Source: CAD feature listing. Evaluate the final solid. Frame: model axes, mm. A direction names the side the tool comes from. Coordinates: 2 decimals unless noted, no trailing zeros. Write each loop counter-clockwise with the first axis right and the second up, starting at its lowest first coordinate (ties: lowest second). Pieces come first, ordered by that corner, then holes. Notation, with made-up numbers: (62, 5) - (80, 5) arc R27 cw to (80, 29) - close; hole circle Ø11 at (29, 59). An arc over 180 degrees is marked (long way). One line per item, written item: value.
from build123d import *

# Parameters (mm, degrees)
CROQUIS1_R              = 1.5
CROQUIS1_W              = 23
CROQUIS1_H              = 10.5
CROQUIS1_R_2            = 1.55
CROQUIS1_W_2            = 8
CROQUIS1_H_2            = 24
SALIENTE_EXTRUIR1_DEPTH = 1


with BuildPart() as part:
    # Croquis1 → Saliente-Extruir1 (new body)
    with BuildSketch(Plane.XY):
        with BuildLine():
            ThreePointArc((309.850726744, 63.509654663), (309.599394258, 62.624115136), (309.514659431, 61.707508197))
            Line((309.514659431, 61.707508197), (309.514659431, 57.327552176))
            ThreePointArc((309.514659431, 57.327552176), (303.729213281, 45.491505651), (290.835726452, 42.785700432))
            ThreePointArc((290.835726452, 42.785700432), (280.128411441, 45.991903753), (269.737322706, 50.109136972))
            ThreePointArc((269.737322706, 50.109136972), (267.74260814, 50.759780707), (265.656038098, 50.97989188))
            Line((265.656038098, 50.97989188), (241.08166038, 50.97989188))
            ThreePointArc((241.08166038, 50.97989188), (235.230334816, 49.089268499), (231.591539837, 44.13228971))
            ThreePointArc((231.591539837, 44.13228971), (233.256794927, -20.949922712), (276.095054953, -69.973905885))
            ThreePointArc((276.095054953, -69.973905885), (277.267588571, -70.441900659), (278.519966502, -70.601286078))
            Line((278.519966502, -70.601286078), (293.924380078, -70.601286078))
            Line((293.924380078, -70.601286078), (366.696152251, -70.601286078))
            ThreePointArc((366.696152251, -70.601286078), (367.948530182, -70.441900659), (369.121063801, -69.973905885))
            ThreePointArc((369.121063801, -69.973905885), (412.002341733, -20.83942385), (413.549540259, 44.357259338))
            ThreePointArc((413.549540259, 44.357259338), (409.908538666, 49.29800924), (404.067243855, 51.18140435))
            Line((404.067243855, 51.18140435), (380.008708846, 51.18140435))
            ThreePointArc((380.008708846, 51.18140435), (377.904907933, 50.95760104), (375.895274543, 50.296208695))
            ThreePointArc((375.895274543, 50.296208695), (365.751190215, 46.2242243), (355.299933141, 43.021923672))
            ThreePointArc((355.299933141, 43.021923672), (342.343405641, 45.666690288), (336.514525798, 57.536423018))
            Line((336.514525798, 57.536423018), (336.514525798, 61.707508197))
            ThreePointArc((336.514525798, 61.707508197), (336.429790971, 62.624115136), (336.178458485, 63.509654663))
            ThreePointArc((336.178458485, 63.509654663), (323.014592614, 72.53553857), (309.850726744, 63.509654663))
        make_face()
        with Locations((256.640896295, -50.101286078)):
            Circle(CROQUIS1_R, mode=Mode.SUBTRACT)
        with Locations((293.924380078, -67.101286078)):
            Circle(CROQUIS1_R, mode=Mode.SUBTRACT)
        with BuildLine():
            Line((287.201459209, -57.50788535), (267.201459209, -57.50788535))
            ThreePointArc((267.201459209, -57.50788535), (277.201459209, -47.50788535), (287.201459209, -57.50788535))
        make_face(mode=Mode.SUBTRACT)
        Polygon((259.608059377, -32.937061776), (253.608059377, -32.937061776), (253.608059377, -12.437061776), (265.608059377, -12.437061776), (265.608059377, -32.937061776), align=None, mode=Mode.SUBTRACT)
        with BuildLine():
            Line((250.731722484, 10.184978786), (250.731722484, -19.815021214))
            Line((250.731722484, -19.815021214), (238.731722484, -19.815021214))
            ThreePointArc((238.731722484, -19.815021214), (238.55388558, -2.343886452), (250.731722484, 10.184978786))
        make_face(mode=Mode.SUBTRACT)
        with Locations((260.608059377, -4.351286077)):
            Circle(CROQUIS1_R, mode=Mode.SUBTRACT)
        with BuildLine():
            ThreePointArc((301.108080537, -22.687061776), (304.239766137, -32.687061776), (301.108080537, -42.687061776))
            Line((301.108080537, -42.687061776), (272.308080537, -42.687061776))
            ThreePointArc((272.308080537, -42.687061776), (269.176394936, -32.687061776), (272.308080537, -22.687061776))
            ThreePointArc((272.308080537, -22.687061776), (286.708080537, -18.980626962), (301.108080537, -22.687061776))
        make_face(mode=Mode.SUBTRACT)
        with Locations((311.80644959, -22.701286077)):
            Circle(CROQUIS1_R, mode=Mode.SUBTRACT)
        with Locations((322.608059377, -22.701286077)):
            Circle(CROQUIS1_R, mode=Mode.SUBTRACT)
        with Locations((311.80644959, -16.851286077)):
            Circle(CROQUIS1_R, mode=Mode.SUBTRACT)
        with Locations((322.608059377, -16.851286077)):
            Circle(CROQUIS1_R, mode=Mode.SUBTRACT)
        with BuildLine():
            Line((331.039483308, -59.416197143), (322.608059377, -67.00788535))
            Line((322.608059377, -67.00788535), (314.115647223, -59.484458572))
            Line((314.115647223, -59.484458572), (308.293872865, -60.935989946))
            Line((308.293872865, -60.935989946), (305.497908348, -56.790802083))
            ThreePointArc((305.497908348, -56.790802083), (297.524016311, -57.967163869), (290.57468702, -62.050496292))
            ThreePointArc((290.57468702, -62.050496292), (296.700568728, -48.781397839), (309.575833339, -41.865983052))
            Line((309.575833339, -41.865983052), (317.608059377, -45.629378016))
            ThreePointArc((317.608059377, -45.629378016), (317.926050133, -44.19732179), (318.644984002, -42.91863604))
            Line((318.644984002, -42.91863604), (318.642820451, -42.911559385))
            Line((318.642820451, -42.911559385), (317.961360482, -40.68260426))
            Line((317.961360482, -40.68260426), (320.108059377, -42.359789251))
            Line((320.108059377, -42.359789251), (322.608059377, -42.359789251))
            Line((322.608059377, -42.359789251), (325.108059377, -42.359789251))
            Line((325.108059377, -42.359789251), (327.254758271, -40.68260426))
            Line((327.254758271, -40.68260426), (326.573298302, -42.911559385))
            Line((326.573298302, -42.911559385), (326.571134752, -42.91863604))
            ThreePointArc((326.571134752, -42.91863604), (327.29006862, -44.19732179), (327.608059377, -45.629378016))
            Line((327.608059377, -45.629378016), (334.361262908, -41.934506878))
            ThreePointArc((334.361262908, -41.934506878), (348.087721137, -48.396503366), (354.701459209, -62.050496292))
            ThreePointArc((354.701459209, -62.050496292), (347.70490498, -57.902513314), (339.657222183, -56.722540654))
            Line((339.657222183, -56.722540654), (336.861257666, -60.867728516))
            Line((336.861257666, -60.867728516), (331.039483308, -59.416197143))
        make_face(mode=Mode.SUBTRACT)
        with Locations((351.291980078, -67.101286078)):
            Circle(CROQUIS1_R, mode=Mode.SUBTRACT)
        with BuildLine():
            ThreePointArc((358.014659544, -57.50788535), (368.014659544, -47.50788535), (378.014659544, -57.50788535))
            Line((378.014659544, -57.50788535), (358.014659544, -57.50788535))
        make_face(mode=Mode.SUBTRACT)
        with Locations((388.037027296, -50.101286078)):
            Circle(CROQUIS1_R, mode=Mode.SUBTRACT)
        with Locations((322.608059377, -32.75788535)):
            Rectangle(CROQUIS1_W, CROQUIS1_H, mode=Mode.SUBTRACT)
        with Locations((333.505439463, -22.701286077)):
            Circle(CROQUIS1_R, mode=Mode.SUBTRACT)
        with BuildLine():
            ThreePointArc((372.908059377, -22.687061776), (376.039744977, -32.687061776), (372.908059377, -42.687061776))
            Line((372.908059377, -42.687061776), (344.108059377, -42.687061776))
            ThreePointArc((344.108059377, -42.687061776), (340.976373776, -32.687061776), (344.108059377, -22.687061776))
            ThreePointArc((344.108059377, -22.687061776), (358.508059377, -18.980624104), (372.908059377, -22.687061776))
        make_face(mode=Mode.SUBTRACT)
        with Locations((333.505439463, -16.851286077)):
            Circle(CROQUIS1_R, mode=Mode.SUBTRACT)
        Polygon((391.608059377, -12.437061776), (391.608059377, -22.687061776), (391.608059377, -32.937061776), (379.608059377, -32.937061776), (379.608059377, -12.437061776), align=None, mode=Mode.SUBTRACT)
        with Locations((384.608059377, -4.351286077)):
            Circle(CROQUIS1_R_2, mode=Mode.SUBTRACT)
        with BuildLine():
            Line((406.484396269, -19.815021214), (394.484396269, -19.815021214))
            Line((394.484396269, -19.815021214), (394.484396269, 10.184978786))
            ThreePointArc((394.484396269, 10.184978786), (406.662233173, -2.343886452), (406.484396269, -19.815021214))
        make_face(mode=Mode.SUBTRACT)
        with Locations((230.456351063, 11.398713923)):
            Circle(CROQUIS1_R, mode=Mode.SUBTRACT)
        with Locations((260.608059377, 3.648713923)):
            Circle(CROQUIS1_R, mode=Mode.SUBTRACT)
        with Locations((260.608059377, 11.648713923)):
            Circle(CROQUIS1_R, mode=Mode.SUBTRACT)
        with Locations((237.850066081, 29.559654286)):
            Circle(CROQUIS1_R, mode=Mode.SUBTRACT)
        with Locations((231.787888255, 33.059654286)):
            Circle(CROQUIS1_R, mode=Mode.SUBTRACT)
        with BuildLine():
            Line((250.471865132, 50.372923914), (251.232957867, 49.522248793))
            Line((251.232957867, 49.522248793), (251.259201082, 33.620640627))
            Line((251.259201082, 33.620640627), (297.835307665, 33.620640627))
            Line((297.835307665, 33.620640627), (308.701459209, 33.620640627))
            ThreePointArc((308.701459209, 33.620640627), (309.439297107, 29.02161934), (308.701459209, 24.422598054))
            Line((308.701459209, 24.422598054), (297.851166076, 24.450299737))
            Line((297.851166076, 24.450299737), (263.676874646, 24.450299737))
            Line((263.676874646, 24.450299737), (263.676874646, 13.478905654))
            Line((263.676874646, 13.478905654), (253.424580574, 24.937918602))
            Line((253.424580574, 24.937918602), (237.324768948, 9.334151374))
            Line((237.324768948, 9.334151374), (250.471865132, 50.372923914))
        make_face(mode=Mode.SUBTRACT)
        with Locations((311.80644959, 24.148694548)):
            Circle(CROQUIS1_R, mode=Mode.SUBTRACT)
        with Locations((322.608059377, 24.148694548)):
            Circle(CROQUIS1_R, mode=Mode.SUBTRACT)
        with Locations((311.80644959, 29.998694548)):
            Circle(CROQUIS1_R, mode=Mode.SUBTRACT)
        with Locations((322.608059377, 29.998694548)):
            Circle(CROQUIS1_R, mode=Mode.SUBTRACT)
        with BuildLine():
            Line((279.812541184, 36.57695454), (253.593005368, 36.514981952))
            Line((253.593005368, 36.514981952), (253.484647579, 46.913395819))
            ThreePointArc((253.484647579, 46.913395819), (268.789341464, 47.197860479), (279.812541184, 36.57695454))
        make_face(mode=Mode.SUBTRACT)
        Polygon((272.608059377, 21.148713923), (283.608059377, 21.148713923), (361.608059377, 21.148713923), (372.608059377, 21.148713923), (375.108059377, 21.148713923), (375.108059377, -13.851286077), (372.908059377, -13.851286077), (272.308059377, -13.851286077), (270.108059377, -13.851286077), (270.108059377, 21.148713923), (272.308059377, 21.148713923), align=None, mode=Mode.SUBTRACT)
        with Locations((333.505439463, 24.148694548)):
            Circle(CROQUIS1_R, mode=Mode.SUBTRACT)
        with Locations((333.505439463, 29.998694548)):
            Circle(CROQUIS1_R, mode=Mode.SUBTRACT)
        with Locations((384.608059377, 3.648713923)):
            Circle(CROQUIS1_R, mode=Mode.SUBTRACT)
        with Locations((384.608059377, 11.648713923)):
            Circle(CROQUIS1_R_2, mode=Mode.SUBTRACT)
        with Locations((414.221552147, 11.398713923)):
            Circle(CROQUIS1_R, mode=Mode.SUBTRACT)
        with BuildLine():
            Line((394.151405418, 33.500405421), (394.207881843, 50.443807073))
            Line((394.207881843, 50.443807073), (394.707680127, 51.065310079))
            Line((394.707680127, 51.065310079), (408.044946606, 9.190500601))
            Line((408.044946606, 9.190500601), (391.971417025, 24.821339763))
            Line((391.971417025, 24.821339763), (381.699853342, 13.379596408))
            Line((381.699853342, 13.379596408), (381.718316867, 24.350974954))
            Line((381.718316867, 24.350974954), (347.544073829, 24.40848614))
            Line((347.544073829, 24.40848614), (336.693749442, 24.399044223))
            ThreePointArc((336.693749442, 24.399044223), (335.972891899, 29.000846221), (336.728676512, 33.597041043))
            Line((336.728676512, 33.597041043), (347.575364789, 33.578787357))
            Line((347.575364789, 33.578787357), (394.151405418, 33.500405421))
        make_face(mode=Mode.SUBTRACT)
        with Locations((407.098258666, 29.672214925)):
            Circle(CROQUIS1_R, mode=Mode.SUBTRACT)
        with Locations((413.160436493, 33.172214925)):
            Circle(CROQUIS1_R, mode=Mode.SUBTRACT)
        with Locations((323.014659431, 53.53553857)):
            Rectangle(CROQUIS1_W_2, CROQUIS1_H_2, mode=Mode.SUBTRACT)
        with BuildLine():
            Line((391.731471174, 46.913395819), (391.623113385, 36.514981952))
            Line((391.623113385, 36.514981952), (365.403577569, 36.57695454))
            ThreePointArc((365.403577569, 36.57695454), (376.426777289, 47.197860479), (391.731471174, 46.913395819))
        make_face(mode=Mode.SUBTRACT)
    extrude(amount=SALIENTE_EXTRUIR1_DEPTH)


solid = part.part
1) Contact query for flat-ended pins moving along their axis: P1, Ø4, axis at x = 260.61, y = -4.35, coming from the -Z side; P2, Ø1.8, axis at x = 414.22, y = 11.4, coming from the +Z side; P3, Ø0.5, axis at x = 284, z = 0.5, coming from the +Y side. Output: stop coordinate, or through.
Values found:
P1: z = 0
P2: through
P3: y = 44.79
2) Material intervals for line 1 (X direction, y = 61, z = 0.85); line 2 (Y direction, x = 329.5, z = 0.8); line 3 (Y direction, x = 317, z = 0.9), sorted ascending.
Values found:
line 1: 309.51 to 319.01, 327.01 to 336.51
line 2: -70.6 to -60.8, -44.59 to -38.01, -27.51 to -13.85, 21.15 to 70.96
line 3: -70.6 to -62.04, -45.34 to -38.01, -27.51 to -13.85, 21.15 to 71.19
3) Section query A-A on y = -10. Output: boundary loops of the cut face in (x, z).
Values found:
outline: (229.73, 0) - (236.93, 0) - (236.93, 1) - (229.73, 1) - close; (250.73, 0) - (270.11, 0) - (270.11, 1) - (250.73, 1) - close; (375.11, 0) - (394.48, 0) - (394.48, 1) - (375.11, 1) - close; (408.29, 0) - (415.49, 0) - (415.49, 1) - (408.29, 1) - close
4) Reachability of faces 1 (the cylindrical face through (280.28, 45.94, 0.49)), 2 (the flat face through (313.536, -43.721, 0.493)), 3 (the cylindrical face through (411.66, -21.71, 0.49)) from +Z, -Z, +X, -X, +Y, -Y: full face, straight path, thin tool, end or side. Return the list, or none.
Values found:
face 1: +Z, -Z, +Y
face 2: +Z, -Z
face 3: +Z, -Z, +X
5) Draft query along Y for faces 4 (the cylindrical face through (365.895, 46.275, 0.493)), 5 (the cylindrical face through (232.923, -20.082, 0.493)), 6 (the flat face through (330.937, -43.808, 0.493)). Return one class per face: released by +Y, released by -Y, zero draft, split by the parting line, or undercut.
Values found:
face 4: released by +Y
face 5: split by the parting line
face 6: undercut
6) Section query B-B on z = 0.75. State how many separate pieces and enclosed holes the cut face has, then the cut area to 3 significant figures.
Values found:
separate pieces: 1
enclosed holes: 44
area: 10,500 mm2
